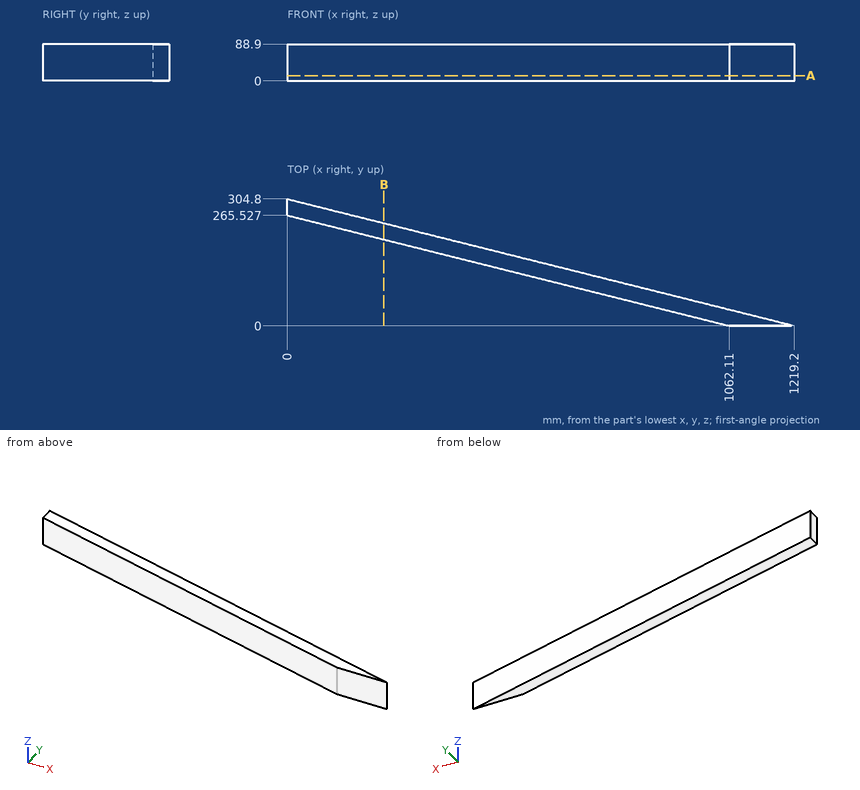
Geometry: see drawing. Coordinates: mm, zero at the bounding-box minimum. Round coordinates to 2 decimals unless told otherwise and drop trailing zeros. Order: outer loops, then holes, each group sorted by start corner. A loop starts at its lowest first (then second) coordinate and runs counter-clockwise, first axis right, second up. Notation, with made-up numbers: (-31.5, 26.5) -> (-6.5, 26.5) arc R23 ccw to (-6.5, 50.5) -> close; hole circle Ø6 at (28.5, 50). An arc over 180 degrees is marked (long way). Answer as CSV lines item,"result".
Item 1: Line query: L1, parallel to Y at x = 343.5, z = 70.5 (1 decimal); L2, parallel to Y at x = 803.5, z = 82.5 (1 decimal). Output: solid intervals per line, ascending.
A:
L1,"179.7 to 218.9"
L2,"64.7 to 103.9"
Item 2: Section B-B, the plane x = 232. Return loops of the section in (y, z), plus the area to 3 significant figures.
A:
outline,"(207.53, 0) -> (246.8, 0) -> (246.8, 88.9) -> (207.53, 88.9) -> close"
area,"3,490 mm²"
Item 3: Section A-A, the plane z = 13. Return loops of the section in (x, y).
A:
outline,"(0, 265.53) -> (1062.11, 0) -> (1219.2, 0) -> (0, 304.8) -> close"
Item 4: Pin query (flat end, axial travel): pin 1 Ø2 at (x, z) = (980.5, 67.5) entering from -Y; pin 2 Ø10 at (x, z) = (519.5, 38.5) entering from +Y (1 decimal). Return the tip coordinate at first contact, or that it passes through.
A:
pin 1,"y = 20.15"
pin 2,"y = 176.2"
